Study the drawing (mm; zero at the part's minimum x, y, z) and answer. Coordinates: 2 decimals unless noted, no trailing zeros. Loops run counter-clockwise (first coordinate to the right, second up) from the corner with the lowest first, then second, coordinate; pieces in that order, holes last. Notation, with made-up numbers: (31, 86.25) -> (77, 86.25) arc R15 cw to (77, 106.25) -> close; hole circle Ø1 at (68, 71). An arc over 180 degrees is marked (long way). One line per question, with ' | ' between items.
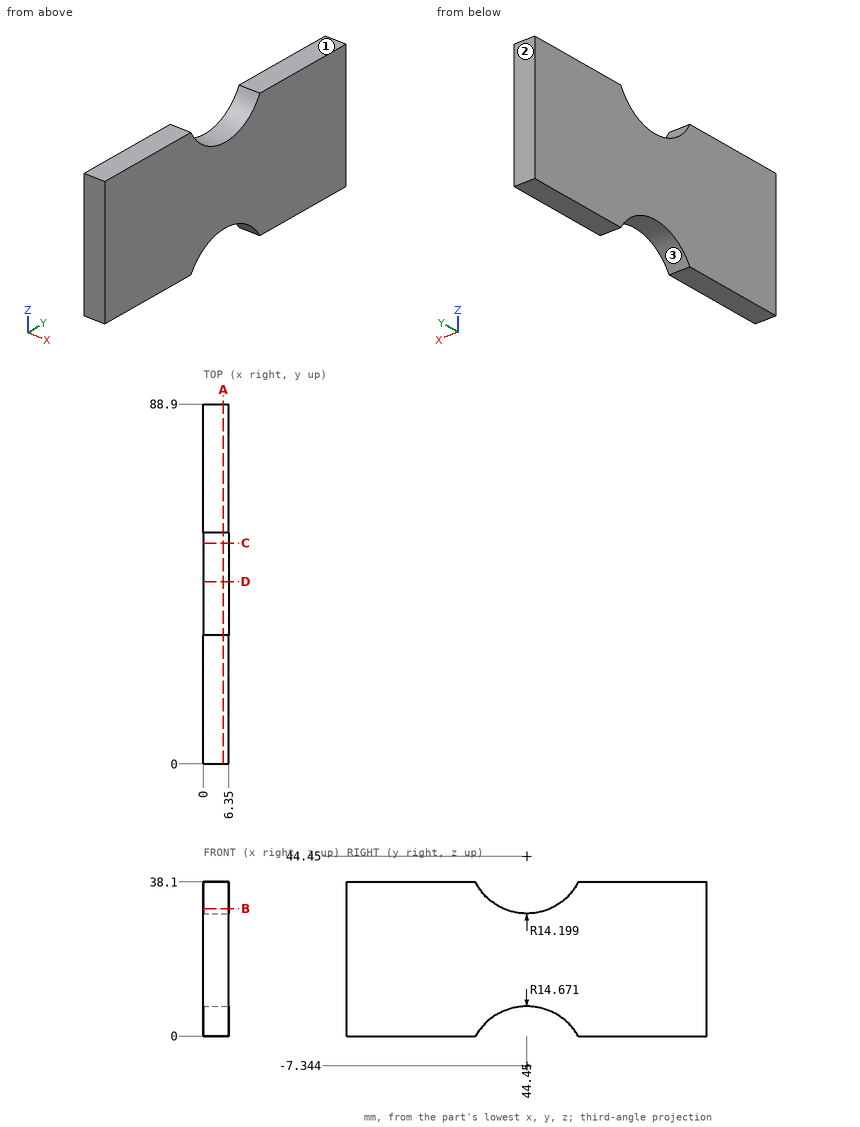
1) The mould has two halves that part along Y. Classify the marked faces 1, 2 and 3: released by +Y, released by -Y, zero draft, split by the parting line, or undercut.
Check values:
face 1: zero draft | face 2: released by +Y | face 3: undercut
2) Find section B-B (z = 31.5). Write down the section's boundary in (x, y).
Check values:
outline: (0, 0) -> (6.35, 0) -> (6.35, 38.63) -> (0, 38.63) -> close; (0, 50.27) -> (6.35, 50.27) -> (6.35, 88.9) -> (0, 88.9) -> close
3) Find section A-A (x = 5). Write down the section's boundary in (y, z).
Check values:
outline: (0, 0) -> (31.75, 0) arc R14.67 cw to (57.15, 0) -> (88.9, 0) -> (88.9, 38.1) -> (57.15, 38.1) arc R14.2 cw to (31.75, 38.1) -> (0, 38.1) -> close
4) Find section D-D (y = 45). Write down the section's boundary in (x, z), plus the area to 3 significant figures.
Check values:
outline: (0, 7.32) -> (6.35, 7.32) -> (6.35, 30.26) -> (0, 30.26) -> close | area: 146 mm^2
5) Find section C-C (y = 54.5). Write down the section's boundary in (x, z).
Check values:
outline: (0, 3.34) -> (6.35, 3.34) -> (6.35, 34.42) -> (0, 34.42) -> close
6) Find the intervals of material crossed by line 1 along Y through (x, z) = (4.25, 35.5) (1 decimal); line 2 along Y through (x, z) = (0.5, 5) (1 decimal); line 3 along Z through (x, y) = (0.5, 48), in increasing order.
Check values:
line 1: y = 0 to 33.4, 55.5 to 88.9 | line 2: y = 0 to 36.5, 52.4 to 88.9 | line 3: z = 6.89 to 30.7
